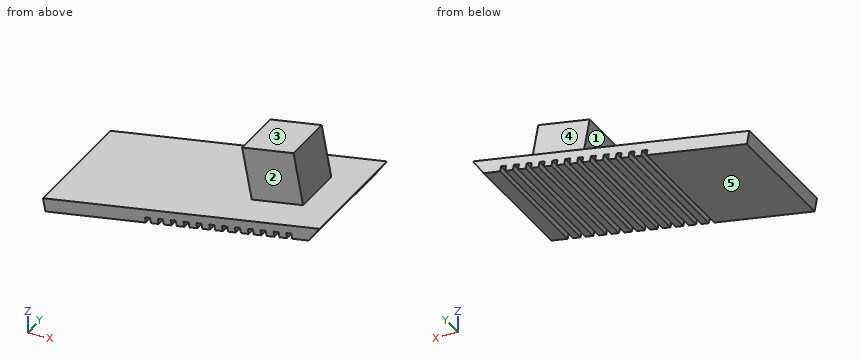
```python
from build123d import *

# Parameters (mm, degrees)
SKETCH1_W           = 56.247710146
SKETCH1_H           = 24
BOSS_EXTRUDE1_DEPTH = 2.54
CHAMFER1_SIZE       = 5
SKETCH2_W           = 1
SKETCH2_H           = 24
CUT_EXTRUDE1_DEPTH  = 1
LPATTERN1_COUNT     = 12
LPATTERN1_PITCH     = 2.5
SKETCH3_W           = 10
SKETCH3_H           = 10
BOSS_EXTRUDE2_DEPTH = 10


with BuildPart() as part:
    # Sketch1 → Boss-Extrude1 (new body)
    with BuildSketch(Plane(origin=(376.193568869, 0, -2012.574360527), x_dir=(-0.9829750210853586, 0, -0.183739238929084), z_dir=(0.183739238929084, 0, -0.9829750210853586))):
        with Locations((-961.949517112, 483.716935274)):
            Rectangle(SKETCH1_W, SKETCH1_H)
    extrude(amount=BOSS_EXTRUDE1_DEPTH)

    # Chamfer1
    # the kernel refuses this chamfer: 5 mm, written as the material it takes off along each edge
    with BuildSketch(Plane(origin=(1349.877660436, 508.575350214, -1833.155789191), x_dir=(-0.15664201033904618, 0, 0.987655446295388), z_dir=(0, -1, 0))) as chamfer1_piece_1:
        Polygon((CHAMFER1_SIZE * 0.999621916911, CHAMFER1_SIZE * 0.0274958766106), (-CHAMFER1_SIZE * 0.0274958766106, CHAMFER1_SIZE * 0.999621916911), (0, 0), align=None)
    extrude(amount=49.71682988, mode=Mode.SUBTRACT)

    # Sketch2 → Cut-Extrude1 (cut)
    with BuildSketch(Plane(origin=(376.660266536, 0, -2015.07111708), x_dir=(-0.9829750210853584, 0, -0.18373923892908509), z_dir=(0.18373923892908506, 0, -0.9829750210853583))):
        with Locations((-981.377561484, 483.716935274)):
            Rectangle(SKETCH2_W, SKETCH2_H)
    cut_extrude1 = extrude(amount=-CUT_EXTRUDE1_DEPTH, mode=Mode.SUBTRACT)

    # LPattern1: Cut-Extrude1 ×12
    with Locations(*[Vector(-0.9829750210853567, 0, -0.18373923892909338) * (i * LPATTERN1_PITCH) for i in range(1, LPATTERN1_COUNT)]):
        add(cut_extrude1, mode=Mode.SUBTRACT)

    # Sketch3 → Boss-Extrude2 (add)
    with BuildSketch(Plane(origin=(376.193568869, 0, -2012.574360527), x_dir=(0.9829750210853584, 0, 0.18373923892908509), z_dir=(-0.18373923892908506, 0, 0.9829750210853583))):
        with Locations((975.613372185, 483.716935274)):
            Rectangle(SKETCH3_W, SKETCH3_H)
    extrude(amount=BOSS_EXTRUDE2_DEPTH)


solid = part.part
```
The listing builds one solid part. Answer for the finished solid, in the listing's coordinates (mm). Face numbers are marked on the shaded views. A direction names the side the tool comes from. Give positions to 0.01 mm unless a question says otherwise; leave off trailing zeros. Write each loop counter-clockwise with the first axis right and the second up, starting at its lowest first coordinate (ties: lowest second). Pieces come first, ordered by that corner, then holes. Notation, with made-up numbers: (7.25, 47) - (44.25, 47) arc R19 cw to (44.25, 76) - close; hole circle Ø10 at (2, -5.5). An arc over 180 degrees is marked (long way). Use one line per item in the form item = value. Start each with the question number.
1) Consider line 1 along Y through (x, z) = (1337.5, -1828.75); line 2 along Z through (x, y) = (1326.5, 489.5); line 3 along Z through (x, y) = (1301, 484.5). Determine where each line is inside the solid, lowest interval first. Write a range as from..to.
2) Find section A-A on z = -1825. Determine the outline of the cut face in (x, y).
3) The mould has two halves that part along Z. Classify the marked faces 1, 2 and 3: pulls with the +Z half, pulls with the -Z half, needs draft (parallel to the pull), parting line crosses it, or undercut.
4) Flat-ended cylindrical pins translate along their axes: pin 1 Ø8 at (x, z) = (1340.5, -1837.5) entering from -Y; pin 2 Ø5 at (y, z) = (479.5, -1826) entering from -X; pin 3 Ø12 at (y, z) = (481.5, -1829) entering from +X; pin 4 Ø8 at (x, y) = (1310, 490) entering from +Z. Find the tip coordinate at first contact, or state that the pin passes through.
5) A tool of negligible diameter and unlimited length cuts with its end or side. For the marked faces 4 and 5, from which of +Z, -Z, +X, -X, +Y, -Y can it reach the whole face along a straight path? Write none if from no direction.
6) Find section B-B on x = 1312. Determine the outline of the cut face in (y, z).
Geometry results:
q1.line_1 = 478.72..488.72
q1.line_2 = -1836.51..-1834.94
q1.line_3 = -1842.29..-1839.71
q2.outline = (1328.56, 478.72) - (1338.73, 478.72) - (1338.73, 488.72) - (1328.56, 488.72) - close
q3.face_1 = undercut
q3.face_2 = needs draft
q3.face_3 = pulls with the +Z half
q4.pin_1 = 471.72
q4.pin_2 = 1328.44
q4.pin_3 = 1346.99
q4.pin_4 = -1837.28
q5.face_4 = +Z, -X, +Y
q5.face_5 = -Z, +X, +Y, -Y
q6.outline = (471.72, -1840.24) - (495.72, -1840.24) - (495.72, -1837.65) - (471.72, -1837.65) - close
